Geometry check sheet. Reference: the model listing, model coordinates, mm. Coordinates: 2 decimals unless noted, no trailing zeros. Loops run counter-clockwise (first coordinate to the right, second up) from the corner with the lowest first, then second, coordinate; pieces in that order, holes last.
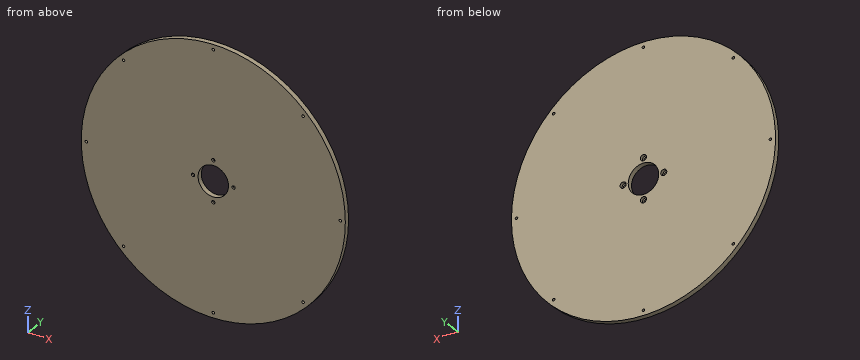
from build123d import *

# Parameters (mm, degrees)
EXTRUDE_1_OUTLINE_R   = 130
EXTRUDE_1_OUTLINE_R_2 = 1.25
EXTRUDE_1_OUTLINE_R_3 = 1.6
EXTRUDE_1_OUTLINE_R_4 = 15
EXTRUDE_1_DEPTH       = 5
SKETCH_2_R            = 3
CUT_EXTRUDE_1_DEPTH   = 3


# Read off the part's stored shape, not the designer's step: ﾎﾞｽ - 押し出し1
with BuildPart() as part:
    # ﾎﾞｽ - 押し出し1 outline → ﾎﾞｽ - 押し出し1 (new body)
    with BuildSketch(Plane(origin=(0, 0, 0), x_dir=(1, 0, 0), z_dir=(0, 1, 0))):
        Circle(EXTRUDE_1_OUTLINE_R)
        with Locations((-88.388347648, -88.388347648)):
            Circle(EXTRUDE_1_OUTLINE_R_2, mode=Mode.SUBTRACT)
        with Locations((0, -125)):
            Circle(EXTRUDE_1_OUTLINE_R_2, mode=Mode.SUBTRACT)
        with Locations((88.388347648, -88.388347648)):
            Circle(EXTRUDE_1_OUTLINE_R_2, mode=Mode.SUBTRACT)
        with Locations((0, -20)):
            Circle(EXTRUDE_1_OUTLINE_R_3, mode=Mode.SUBTRACT)
        with Locations((-125, 0)):
            Circle(EXTRUDE_1_OUTLINE_R_2, mode=Mode.SUBTRACT)
        with Locations((-20, 0)):
            Circle(EXTRUDE_1_OUTLINE_R_3, mode=Mode.SUBTRACT)
        with Locations((-88.388347648, 88.388347648)):
            Circle(EXTRUDE_1_OUTLINE_R_2, mode=Mode.SUBTRACT)
        Circle(EXTRUDE_1_OUTLINE_R_4, mode=Mode.SUBTRACT)
        with Locations((20, 0)):
            Circle(EXTRUDE_1_OUTLINE_R_3, mode=Mode.SUBTRACT)
        with Locations((0, 20)):
            Circle(EXTRUDE_1_OUTLINE_R_3, mode=Mode.SUBTRACT)
        with Locations((125, 0)):
            Circle(EXTRUDE_1_OUTLINE_R_2, mode=Mode.SUBTRACT)
        with Locations((0, 125)):
            Circle(EXTRUDE_1_OUTLINE_R_2, mode=Mode.SUBTRACT)
        with Locations((88.388347648, 88.388347648)):
            Circle(EXTRUDE_1_OUTLINE_R_2, mode=Mode.SUBTRACT)
    extrude(amount=EXTRUDE_1_DEPTH)

    # ｽｹｯﾁ2 → ｶｯﾄ - 押し出し1 (cut)
    with BuildSketch(Plane(origin=(0, 5, 0), x_dir=(1, 0, 0), z_dir=(0, 1, 0))):
        with Locations(Location((0, 20, 0), (0, 0, 270))):
            Circle(SKETCH_2_R)
        with Locations(Location((20, 0, 0), (0, 0, 270))):
            Circle(SKETCH_2_R)
        with Locations(Location((0, -20, 0), (0, 0, 270))):
            Circle(SKETCH_2_R)
        with Locations(Location((-20, 0, 0), (0, 0, 270))):
            Circle(SKETCH_2_R)
    extrude(amount=-CUT_EXTRUDE_1_DEPTH, mode=Mode.SUBTRACT)


solid = part.part
(1) Gauge pin test, flat ends, axial feed: pin 1 Ø5 at (x, z) = (0, -20) entering from +Y; pin 2 Ø3 at (x, z) = (-20, 0) entering from -Y; pin 3 Ø1 at (x, y) = (100, 4) entering from +Z. Record the tip position at first contact, or that the pin passes through.
Findings:
pin 1: stops at y = 2
pin 2: passes through
pin 3: stops at z = 83.66
(2) Sectioned sample at A-A on x = 7.5. Record the cut outline in (y, z), and give its area (3 significant figures).
Findings:
outline: (0, -129.78) - (5, -129.78) - (5, -12.99) - (0, -12.99) - close; (0, 12.99) - (5, 12.99) - (5, 129.78) - (0, 129.78) - close
area: 1,170 mm2
(3) Sectioned sample at B-B on y = 4.2. State how many separate pieces and enclosed holes the cut face has, and give its area (3 significant figures).
Findings:
separate pieces: 1
enclosed holes: 13
area: 52,200 mm2
(4) Sectioned sample at C-C on z = -9. Record the cut outline in (x, y), and give its area (3 significant figures).
Findings:
outline: (-129.69, 0) - (-12, 0) - (-12, 5) - (-129.69, 5) - close; (12, 0) - (129.69, 0) - (129.69, 5) - (12, 5) - close
area: 1,180 mm2
(5) Sectioned sample at D-D on x = 79.5. Record the cut outline in (y, z).
Findings:
outline: (0, -102.86) - (5, -102.86) - (5, 102.86) - (0, 102.86) - close
(6) Scan lines: L1, parallel to Z at x = 0, y = 1.75; L2, parallel to X at y = 2.3, z = -6.5. Record each from-to range of solid material in increasing order.
Findings:
L1: z = -130 to -126.25, -123.75 to -21.6, -18.4 to -15, 15 to 18.4, 21.6 to 123.75, 126.25 to 130
L2: x = -129.84 to -13.52, 13.52 to 129.84
